Here's the drawing with two shaded views (mm, measured from the low corner). I have some questions. A direction names the side the tool comes from. Round coordinates to 2 decimals unless told otherwise and drop trailing zeros. Loops run counter-clockwise (first coordinate to the right, second up) from the corner with the lowest first, then second, coordinate; pieces in that order, holes last. Notation, with made-up numbers: (38.5, 35) -> (64.5, 35) arc R8 ccw to (64.5, 48) -> close; hole circle Ø11 at (19.5, -31). An arc over 180 degrees is marked (long way). Write each question's results on one line, items separated by ' | '. Start each with the question number.
1) Imagine slicing it at B-B, the plane y = 114.3. List the corners of the cut face in (x, z) for me, plus the area to 3 significant figures.
2) Imagine slicing it at D-D, the plane x = 1276. List the corners of the cut face in (y, z) for me.
3) For P1, Ø8, axis at x = 803, y = 99, coming from the +Z side, with a flat end and sliding along its axis, tell me the tip position at first contact or that it passes through.
4) Imagine slicing it at A-A, the plane x = 190.5. List the corners of the cut face in (y, z) for me.
5) If I drill on probe 1 along Z at (x, y) = (774, 69.5); probe 2 along X at (y, z) = (136.5, 285); probe 3 along X at (y, z) = (105.5, 278), over which ranges is the centre line in solid material (lowest first)?
6) Imagine slicing it at C-C, the plane z = 294. List the corners of the cut face in (x, y) for me.
7) We'd pull the mould along X, two halves only. Please class the marked faces 3, 4, 5 and 6: pulls with the +X half, pulls with the -X half, needs draft (parallel to the pull), parting line crosses it, or undercut.
8) Which directions (+Z, -Z, +X, -X, +Y, -Y) give clear straight access to the entire face, cutting with the end or side of a thin tool? Please do the marked faces 1 and 2.
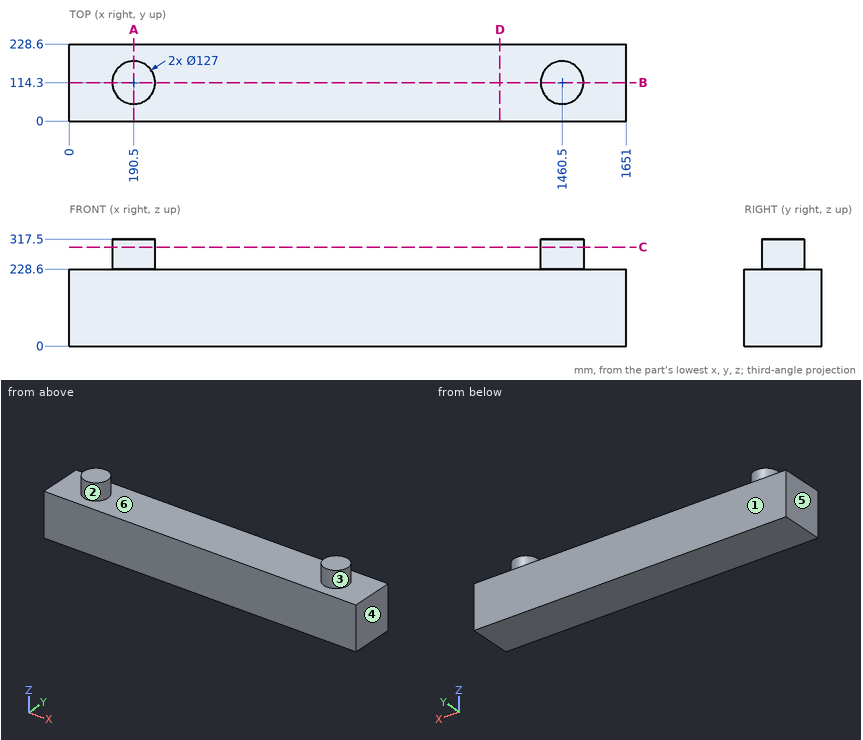
Checked values:
1) outline: (0, 0) -> (1651, 0) -> (1651, 228.6) -> (1524, 228.6) -> (1524, 317.5) -> (1397, 317.5) -> (1397, 228.6) -> (254, 228.6) -> (254, 317.5) -> (127, 317.5) -> (127, 228.6) -> (0, 228.6) -> close | area: 400,000 mm^2
2) outline: (0, 0) -> (228.6, 0) -> (228.6, 228.6) -> (0, 228.6) -> close
3) P1: z = 228.6
4) outline: (0, 0) -> (228.6, 0) -> (228.6, 228.6) -> (177.8, 228.6) -> (177.8, 317.5) -> (50.8, 317.5) -> (50.8, 228.6) -> (0, 228.6) -> close
5) probe 1: 0 to 228.6 | probe 2: 131.01 to 249.99, 1401.01 to 1519.99 | probe 3: 127.61 to 253.39, 1397.61 to 1523.39
6) outline: circle Ø127 at (190.5, 114.3); circle Ø127 at (1460.5, 114.3)
7) face 3: undercut | face 4: pulls with the +X half | face 5: pulls with the -X half | face 6: undercut
8) face 1: +Z, -Z, +X, -X, +Y | face 2: +Z
